Autodesk Inventor part; units mm, degrees
ref_plane "YZ Plane" through (0, 0, 0) normal (1, 0, 0) x (0, 1, 0)
ref_plane "XZ Plane" through (0, 0, 0) normal (0, 1, 0) x (-1, 0, 0)
ref_plane "XY Plane" through (0, 0, 0) normal (0, 0, 1) x (1, 0, 0)
sketch "Esquisse3" plane through (0, 0, 0) normal (0, 1, 0) x (-1, 0, 0)
  line L0 (4, 0) -> (-4, 0)
  line L1 (-4, 0) -> (-4, -30)
  arc A0 (-4, -30) -> (4, -22) centre (-4, -22) ccw
  line L2 (4, 0) -> (4, -22)
  point P0 (0, 0)
  point P1 (0, 0)
  dimension "d21" = 8
  dimension "d22" = 30
extrude "Extrusion2" add sketch "Esquisse3" along normal mid plane 8
sketch "Esquisse4" plane through (0, 0, 0) normal (0, 1, 0) x (-1, 0, 0)
  line L0 (-4, 0) -> (4, 0)
  line L1 (4, 0) -> (4, -22)
  arc A0 (-4, -30) -> (4, -22) centre (-4, -22) ccw
  line L2 (-4, -30) -> (-4, 0)
  line L3 (-4, -30) -> (-4, 0)
  line L4 (-2, -22) -> (-2, 0)
  arc A1 (-4, -24) -> (-2, -22) centre (-4, -22) ccw
  point P0 (0, 0)
  dimension "d26" = 6
  dimension "d27" = 6
extrude "Extrusion3" cut sketch "Esquisse4" along normal mid plane 3 contours L0 L1 A0 L2 A1 L4
sketch "Esquisse5" plane through (0, 4, 0) normal (0, 1, 0) x (1, 0, 0)
  line L0 (4, 30) -> (4, 0)
  line L1 (4, 0) -> (12, 0)
  line L2 (12, 0) -> (12, 8)
  line L3 (12, 8) -> (4, 8)
  line L4 (4, 8) -> (4, 0)
  point P0 (0, 0)
  dimension "d30" = 8
  dimension "d31" = 8
extrude "Extrusion4" add sketch "Esquisse5" against normal up to surface (8 mm away)
sketch "Esquisse6" plane through (0, 4, 0) normal (0, 1, 0) x (1, 0, 0)
  line L0 (-4, 0) -> (12, 0)
  line L1 (12, 0) -> (12, 8)
  line L2 (4, 8) -> (4, 30)
  point P0 (0, 0)
  point P1 (8, 4)
  dimension "d34" = 4
  dimension "d47" = 4
hole "Perçage2" at (8, 4, -4) direction (0, -1, 0) diameter 4 depth 8
fillet "Congé2" radius 1.5 3 edges at (-4, 2.75, 0) (-4, -2.75, 0) (4, 0, -8)
fillet "Congé3" radius 4 2 edges at (12, 0, 0) (12, 0, -8)
sketch "Esquisse7" plane through (-4, 1.5, -22) normal (-1, 0, 0) x (0, 0, 1)
  line L0 (16, 2.5) -> (20, 2.5)
  line L1 (20.5, -5.5) -> (0, -5.5)
  line L2 (20.5, -3) -> (0, -3)
  line L3 (17.5, -5.5) -> (18.5, -5.5)
  line L4 (18.5, -5.5) -> (18.5, -3)
  line L5 (18.5, -3) -> (17.5, -3)
  line L6 (17.5, -3) -> (17.5, -5.5)
  line L7 (0, 0) -> (20.5, 0)
  line L8 (0, 2.5) -> (20.5, 2.5)
  line L9 (17.5, 0) -> (18.5, 0)
  line L10 (18.5, 0) -> (18.5, 2.5)
  line L11 (18.5, 2.5) -> (17.5, 2.5)
  line L12 (17.5, 2.5) -> (17.5, 0)
  line L13 (20, -5.5) -> (16, -5.5)
  line L14 (16, 2.5) -> (20, 2.5)
  point P0 (22, -1.5)
  point P1 (18, 2.5)
  dimension "d49" = 1
extrude "Extrusion5" cut sketch "Esquisse7" against normal blind 1
properties part number "viseur_reglable_piece"
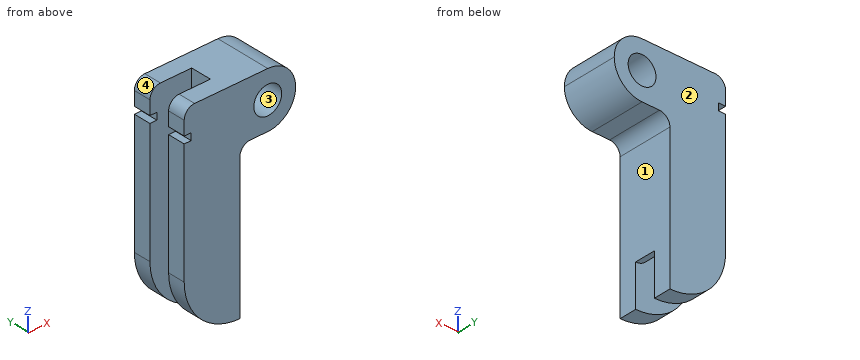
Work out the finished part from the listing and answer in its coordinate system (mm). Face numbers are marked on the shaded views. Round coordinates to 2 decimals unless told otherwise and drop trailing zeros. Write each loop counter-clockwise with the first axis right and the second up, starting at its lowest first coordinate (ties: lowest second). Pieces come first, ordered by that corner, then holes.
1) A cutting plane is placed at C-C (x = -1.5). Give the vertices of the cut face in (y, z).
2) Straight lines are drawn through the part: line 1 (Z direction, x = 8, y = 0); line 2 (X direction, y = -1.75, z = -4); line 3 (X direction, y = -0.25, z = -4). For each, find the intervals that lie inside material, in ascending order.
3) The mould has two halves that part along X. Classify the marked faces 1, 2, 3 and 4: pulls with the +X half, pulls with the -X half, needs draft (parallel to the pull), parting line crosses it, or undercut.
4) Given pin 1 Ø0.9 at (y, z) = (0.5, -14) entering from -X; pin 2 Ø0.8 at (x, y) = (-3.5, 2.5) entering from +Z; pin 3 Ø1.1 at (x, y) = (-3.5, -2.5) entering from -Z, each flat-ended and moving along its own axis, determine where each tip first touches the part or whether it passes through.
5) A cutting plane is placed at B-B (z = -19). Give the vertices of the cut face in (x, y).
6) A cutting plane is placed at D-D (x = 9.25). Give the vertices of the cut face in (y, z).
Completed:
1. outline: (-4, -27.81) - (-1.5, -27.81) - (-1.5, 0) - (-4, 0) - close; (1.5, -27.81) - (4, -27.81) - (4, 0) - (1.5, 0) - close
2. line 1: z = -8 to -6, -2 to 0
2. line 2: x = -3 to 6, 10 to 12
2. line 3: x = 2 to 6, 10 to 12
3. face 1: pulls with the +X half
3. face 2: needs draft
3. face 3: undercut
3. face 4: pulls with the -X half
4. pin 1: stops at x = 2
4. pin 2: stops at z = -0.13
4. pin 3: stops at z = -25.96
5. outline: (-4, -4) - (4, -4) - (4, 4) - (-4, 4) - (-4, 1.5) - (2, 1.5) - (2, -1.5) - (-4, -1.5) - close
6. outline: (-4, -7.8) - (4, -7.8) - (4, -5.56) - (-4, -5.56) - close; (-4, -2.44) - (4, -2.44) - (4, -0.2) - (-4, -0.2) - close
